```python
from build123d import *

# Parameters (mm, degrees)
F0_W          = 225
F0_H          = 270.5
F1_DEPTH      = 30
F2_R          = 3
F3_W          = 30
F3_H          = 76.5
F4_DEPTH      = 3
F5_R          = 2.99999
F6_W          = 21
F6_H          = 238
F7_DEPTH      = 3
F8_R          = 2.99999
F9_W          = 21
F9_H          = 145
F10_DEPTH     = 61
F11_R         = 3
F12_T1_DEPTH  = 28.6800979278
F12_T3_DEPTH  = 28.6800979278
F12_T8_DEPTH  = 15.4301079278
F12_T13_DEPTH = 15.4301079278
F13_W         = 61
F13_H         = 13
F14_DEPTH     = 5
F15_R         = 3
F16_R         = 1
F17_DEPTH     = 25


# Not quite as in the source:
# - a fillet or chamfer that OpenCascade refuses, or shapes differently, is made with other operations: its cross-section is extruded or revolved along the edge and cut away or added
# - a fillet or chamfer is up to 0.001 mm smaller than in the source, because OpenCascade refuses the exact size


with BuildPart() as f1:
    # F0 (on Front) → F1 (new body)
    with BuildSketch(Plane.XZ):
        Rectangle(F0_W, F0_H)
    extrude(amount=F1_DEPTH)

    # F2
    f2_edges = [f1.edges().sort_by_distance(p)[0] for p in [
        (112.5, -15, 135.25),
        (112.5, -15, -135.25),
        (-112.5, -15, 135.25),
        (-112.5, -15, -135.25),
    ]]
    fillet(f2_edges, radius=F2_R)

    # F3 (on face) → F4 (cut)
    with BuildSketch(Plane.YZ.offset(112.5)):
        with Locations((-15, 66.25)):
            Rectangle(F3_W, F3_H)
        with Locations((-15, -66.25)):
            Rectangle(F3_W, F3_H)
    extrude(amount=-F4_DEPTH, mode=Mode.SUBTRACT)

    # F5 (radius 3 in the source; OpenCascade refuses exactly that, so slightly less here)
    f5_edges = [f1.edges().sort_by_distance(p)[0] for p in [
        (109.5, -15, 28),
        (109.5, -15, -104.5),
        (109.5, -15, -28),
        (109.5, -15, 104.5),
    ]]
    fillet(f5_edges, radius=F5_R)

    # F6 (on face) → F7 (cut)
    with BuildSketch(Plane(origin=(-112.5, 0, 0), x_dir=(0, -1, 0), z_dir=(-1, 0, 0))):
        with Locations((10.5, 0)):
            Rectangle(F6_W, F6_H)
    extrude(amount=-F7_DEPTH, mode=Mode.SUBTRACT)

    # F8 (radius 3 in the source; OpenCascade refuses exactly that, so slightly less here)
    f8_edges = [f1.edges().sort_by_distance(p)[0] for p in [
        (-109.5, -10.5, -119),
        (-109.5, -10.5, 119),
    ]]
    fillet(f8_edges, radius=F8_R)

    # F9 (on face) → F10 (cut)
    with BuildSketch(Plane(origin=(-109.5, 0, 0), x_dir=(0, -1, 0), z_dir=(-1, 0, 0))):
        with Locations((10.5, 0)):
            Rectangle(F9_W, F9_H)
    extrude(amount=-F10_DEPTH, mode=Mode.SUBTRACT)

    # F11
    f11_edges = [f1.edges().sort_by_distance(p)[0] for p in [
        (-48.5, -10.5, -72.5),
        (-48.5, -10.5, 72.5),
    ]]
    fillet(f11_edges, radius=F11_R)

    # F12: chamfer of 3 on 6 edges, made by hand

    # F12_s2 → F12_t1 (cut)
    with BuildSketch(Plane.XY.offset(-139.9650489639)):
        Polygon((-109.5, 0), (-112.5, -3), (-112.5, 0), align=None)
    extrude(amount=F12_T1_DEPTH, mode=Mode.SUBTRACT)

    # F12_s4 → F12_t3 (cut)
    with BuildSketch(Plane.XY.offset(111.2849510361)):
        Polygon((-109.5, 0), (-112.5, -3), (-112.5, 0), align=None)
    extrude(amount=F12_T3_DEPTH, mode=Mode.SUBTRACT)


with BuildPart() as f12_tool6:
    # F12_s7 → F12_t8 (new body)
    with BuildSketch(Plane.YZ.offset(-120.2150489639)):
        Polygon((0, -122), (-3, -119), (0, -119), align=None)
    extrude(amount=F12_T8_DEPTH)

    split(bisect_by=Plane(origin=(-54.75, 54.75, 0), x_dir=(0, 0, 1), z_dir=(-0.7071067812, 0.7071067812, 0)), keep=Keep.TOP)


with BuildPart() as f1_1:
    add(f1.part)

    # F12_t5: cut F12_tool6
    add(f12_tool6.part, mode=Mode.SUBTRACT)


with BuildPart() as f12_tool11:
    # F12_s12 → F12_t13 (new body)
    with BuildSketch(Plane.YZ.offset(-120.2150489639)):
        Polygon((0, 122), (-3, 119), (0, 119), align=None)
    extrude(amount=F12_T13_DEPTH)

    split(bisect_by=Plane(origin=(-54.75, 54.75, 0), x_dir=(0, 0, 1), z_dir=(-0.7071067812, 0.7071067812, 0)), keep=Keep.TOP)


with BuildPart() as f1_2:
    add(f1_1.part)

    # F12_t10: cut F12_tool11
    add(f12_tool11.part, mode=Mode.SUBTRACT)

    # F13 (on face) → F14 (cut)
    with BuildSketch(Plane(origin=(0, 0, 0), x_dir=(-1, 0, 0), z_dir=(0, 1, 0))):
        with Locations((79, 76)):
            Rectangle(F13_W, F13_H)
    extrude(amount=-F14_DEPTH, mode=Mode.SUBTRACT)

    # F15
    f15_edges = [f1_2.edges().sort_by_distance(p)[0] for p in [
        (-48.5, -2.5, 82.5),
    ]]
    fillet(f15_edges, radius=F15_R)

    # F16 (on face) → F17 (cut)
    with BuildSketch(Plane.XZ.offset(30)):
        with Locations((-90.5, 75)):
            Circle(F16_R)
        with Locations((-90.5, 27)):
            Circle(F16_R)
    extrude(amount=-F17_DEPTH, mode=Mode.SUBTRACT)


solid = f1_2.part
```
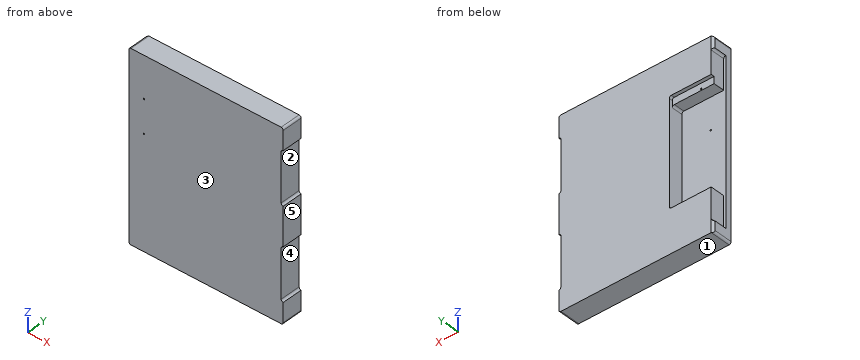
Check sheet for the modelled part. Datum: model origin and axes. Units: mm. Face numbers are marked on the shaded views. A direction names the side the tool comes from. Give positions to 0.01 mm unless a question says otherwise; leave off trailing zeros. Order: outer loops, then holes, each group sorted by start corner. A loop starts at its lowest first (then second) coordinate and runs counter-clockwise, first axis right, second up. Notation, with made-up numbers: M 49,-27.75 L 72,-27.75 A29 cw 72,-1.75 Z; hole C -11.5,18 d2. An arc over 180 degrees is marked long. Answer in a Markdown table with one row per item. Add a question column.
Q1. Access from +Z, -Z, +X, -X, +Y, -Y to the whole of each face (thin tool, end or side, straight path). Record for the marked faces 4 and 5.
Q2. Thickness scan on L1, parallel to Z at x = -90.5, y = -22.5; L2, parallel to X at y = -14, z = 75; L3, parallel to Z at x = -51, y = -8. Record the ranges inside material, lowest first.
Q3. Release check for a two-part mould opening along Z. For the marked faces 1, 2 and 3 record: released by +Z, released by -Z, zero draft, split by the parting line, or undercut.
Q4. Sectioned sample at C-C, the plane z = -54.5. Record the boundary of the cut face in (x, y).
Q5. Gauge pin test, flat ends, axial feed: pin 1 Ø2 at (y, z) = (-8.5, -13.5) entering from -X; pin 2 Ø14.5 at (x, z) = (-74.5, 74.5) entering from +Y; pin 3 Ø19 at (x, z) = (-89.5, -26.5) entering from +Y. Record the tip position at first contact, or that the pin passes through.
Q6. Sectioned sample at B-B, the plane x = -84.5. Record the boundary of the cut face in (y, z).
Verdict:
| question | item | result |
|---|---|---|
| 1 | face 4 | +X, +Y, -Y |
| 1 | face 5 | +Z, -Z, +X, +Y, -Y |
| 2 | L1 | -135.25 to 26, 28 to 74, 76 to 135.25 |
| 2 | L2 | -109.5 to -91.5, -89.5 to 109.5 |
| 2 | L3 | -135.25 to -72.46, 72.46 to 135.25 |
| 3 | face 1 | released by -Z |
| 3 | face 2 | undercut |
| 3 | face 3 | zero draft |
| 4 | outline | M -112.5,-30 L 109.5,-30 L 109.5,0 L -48.5,0 L -48.5,-21 L -112.5,-21 Z |
| 5 | pin 1 | x = -48.5 |
| 5 | pin 2 | y = -5 |
| 5 | pin 3 | y = -21 |
| 6 | outline | M -30,-135.25 L 0,-135.25 L 0,-72.5 L -21,-72.5 L -21,72.5 L -5,72.5 L -5,82.5 L 0,82.5 L 0,135.25 L -30,135.25 Z |
